from build123d import *

# Parameters (mm, degrees)
SKETCH1_W           = 26
SKETCH1_H           = 37.5
SKETCH1_R           = 8
BOSS_EXTRUDE1_DEPTH = 14
SKETCH2_R           = 1.75
CUT_EXTRUDE1_DEPTH  = 32
SKETCH5_R           = 8.35
SKETCH5_R_2         = 6
BOSS_EXTRUDE3_DEPTH = 3
FILLET3_R           = 1


with BuildPart() as part:
    # Sketch1 → Boss-Extrude1 (new, symmetric)
    with BuildSketch(Plane(origin=(0, 0, 0), x_dir=(0, 0, -1), z_dir=(1, 0, 0))):
        Rectangle(SKETCH1_W, SKETCH1_H)
        Circle(SKETCH1_R, mode=Mode.SUBTRACT)
    extrude(amount=BOSS_EXTRUDE1_DEPTH, both=True)

    # Sketch2 → Cut-Extrude1 (cut)
    with BuildSketch(Plane(origin=(0, 18.75, 0), x_dir=(1, 0, 0), z_dir=(0, 1, 0))):
        with Locations(Location((-10, 10, 0), (0, 0, 270))):
            Circle(SKETCH2_R)
        with Locations(Location((10, 10, 0), (0, 0, 270))):
            Circle(SKETCH2_R)
        with Locations(Location((10, -10, 0), (0, 0, 270))):
            Circle(SKETCH2_R)
        with Locations(Location((-10, -10, 0), (0, 0, 270))):
            Circle(SKETCH2_R)
    extrude(amount=-CUT_EXTRUDE1_DEPTH, mode=Mode.SUBTRACT)

    # Sketch5 → Boss-Extrude3 (add)
    with BuildSketch(Plane.ZY.offset(14)):
        Circle(SKETCH5_R)
        Circle(SKETCH5_R_2, mode=Mode.SUBTRACT)
    extrude(amount=-BOSS_EXTRUDE3_DEPTH)

    # Fillet3
    fillet3_edges = [part.edges().sort_by_distance(p)[0] for p in [
        (14, 0, 13),
        (14, 0, -13),
        (-14, 0, 13),
        (-14, 18.75, 0),
        (-14, 0, -13),
        (0, 18.75, 13),
        (0, 18.75, -13),
        (14, 18.75, 0),
    ]]
    fillet(fillet3_edges, radius=FILLET3_R)


solid = part.part
The listing builds one solid part. Answer for the finished solid, in the listing's coordinates (mm). A direction names the side the tool comes from. Give positions to 0.01 mm unless a question says otherwise; leave off trailing zeros. Write each loop counter-clockwise with the first axis right and the second up, starting at its lowest first coordinate (ties: lowest second). Pieces come first, ordered by that corner, then holes. Notation, with made-up numbers: (85.5, -27.75) -> (103.5, -27.75) arc R18 cw to (103.5, -5.75) -> close; hole circle Ø9 at (5, 28). An arc over 180 degrees is marked (long way). One line per question, with ' | ' between items. Start each with the question number.
1. For a pull along X with two mould halves and no side action, classify faces 1 (the flat face through (10, -13.25, -10)), 2 (the cylindrical face through (-13.715, -0.244, 12.699)), 3 (the cylindrical face through (13.699, 18.465, -0.168)) as pulls with the +X half, pulls with the -X half, needs draft (parallel to the pull), parting line crosses it, or undercut.
2. Find the intervals of material crossed by probe 1 along X at (y, z) = (8, 10); probe 2 along Z at (x, y) = (9.5, -4.5); probe 3 along Y at (x, z) = (-12.65, 0), in increasing order.
3. Given pin 1 Ø3 at (x, z) = (-10, -10) entering from +Y; pin 2 Ø1.5 at (y, z) = (6.5, 0) entering from +X, each flat-ended and moving along its own axis, determine where each tip first touches the part or whether it passes through.
4. Section D-D (y = -7) is taken. Determine the outline of the cut face in (x, z), plus the area to 3 significant figures.
5. Section B-B (z = 0) is taken. Determine the outline of the cut face in (x, y).
6. For faces 4 (the flat face through (-11, 6, -2)), 5 (the cylindrical face through (-13.715, -0.244, -12.699)), 6 (the cylindrical face through (-8.5, 3, -9.1)), determine the directions among +Z, -Z, +X, -X, +Y, -Y from which every point of the face is accessible in a straight line to the end or side of a thin tool.
7. Section C-C (x = -3.5) is taken. Determine the outline of the cut face in (y, z).
8. Section A-A (y = -0.5) is taken. Determine the outline of the cut face in (x, z), plus the area to 3 significant figures.
Response values:
1) face 1: undercut | face 2: pulls with the -X half | face 3: pulls with the +X half
2) probe 1: -14 to -11.75, -8.25 to 8.25, 11.75 to 14 | probe 2: -13 to -11.68, -8.32 to -6.61, 6.61 to 8.32, 11.68 to 13 | probe 3: -18.75 to -6, 6 to 18.75
3) pin 1: y = -13.25 | pin 2: x = -11
4) outline: (-14, -12) arc R1 ccw to (-13, -13) -> (13, -13) arc R1 ccw to (14, -12) -> (14, -3.87) -> (-11, -3.87) -> (-11, 3.87) -> (14, 3.87) -> (14, 12) arc R1 ccw to (13, 13) -> (-13, 13) arc R1 ccw to (-14, 12) -> close; hole circle Ø3.5 at (-10, -10); hole circle Ø3.5 at (-10, 10); hole circle Ø3.5 at (10, -10); hole circle Ø3.5 at (10, 10) | area: 495 mm2
5) outline: (-14, -18.75) -> (14, -18.75) -> (14, -8) -> (-11, -8) -> (-11, -6) -> (-14, -6) -> close; (-14, 6) -> (-11, 6) -> (-11, 8) -> (14, 8) -> (14, 17.75) arc R1 ccw to (13, 18.75) -> (-13, 18.75) arc R1 ccw to (-14, 17.75) -> close
6) face 4: +X | face 5: -Z, -X, +Y, -Y | face 6: +Y
7) outline: (-18.75, -13) -> (17.75, -13) arc R1 ccw to (18.75, -12) -> (18.75, 12) arc R1 ccw to (17.75, 13) -> (-18.75, 13) -> close; hole circle Ø16 at (0, 0)
8) outline: (-14, -12) arc R1 ccw to (-13, -13) -> (13, -13) arc R1 ccw to (14, -12) -> (14, -7.98) -> (-11, -7.98) -> (-11, -5.98) -> (-14, -5.98) -> close; (-14, 5.98) -> (-11, 5.98) -> (-11, 7.98) -> (14, 7.98) -> (14, 12) arc R1 ccw to (13, 13) -> (-13, 13) arc R1 ccw to (-14, 12) -> close; hole circle Ø3.5 at (-10, -10); hole circle Ø3.5 at (-10, 10); hole circle Ø3.5 at (10, -10); hole circle Ø3.5 at (10, 10) | area: 254 mm2
